```python
from build123d import *

# Parameters (mm, degrees)
F1_DEPTH  = 15
F2_W      = 3
F2_H      = 296.3
F3_DEPTH  = 25
F4_R      = 2.5
F5_DEPTH  = 3
F6_W      = 1
F6_H      = 0.5
F7_DEPTH  = 3
F8_R      = 1
F9_R      = 2.5
F9_R_2    = 1.2
F10_DEPTH = 3
F11_R     = 1.2
F12_DEPTH = 34.2
F13_DEPTH = 3
F14_R     = 2


with BuildPart() as f1:
    # F0 (on Right) → F1 (new body)
    with BuildSketch(Plane.YZ):
        Polygon((-7.5968508422, 3), (-7.5968508422, 0), (22.4031491578, 0), (22.4031491578, 304.3), (19.4031491578, 304.3), (19.4031491578, 3), align=None)
    extrude(amount=F1_DEPTH)

    # F2 (on face) → F3 (join)
    with BuildSketch(Plane(origin=(0, 22.4031491578, 0), x_dir=(-1, 0, 0), z_dir=(0, 1, 0))):
        with Locations((1.5, 156.15)):
            Rectangle(F2_W, F2_H)
        with Locations((-16.5, 156.15)):
            Rectangle(F2_W, F2_H)
    extrude(amount=-F3_DEPTH)

    # F4 (on face) → F5 (cut)
    with BuildSketch(Plane.XY.offset(3)):
        with Locations((7.5, -2.5968508422)):
            Circle(F4_R)
        with Locations((7.5, 12.4031491578)):
            Circle(F4_R)
    extrude(amount=-F5_DEPTH, mode=Mode.SUBTRACT)

    # F6 (on face) → F7 (cut)
    with BuildSketch(Plane.XZ.offset(-19.4031491578)):
        with Locations((0.5, 7.75)):
            Rectangle(F6_W, F6_H)
        with Locations((14.5, 7.75)):
            Rectangle(F6_W, F6_H)
    extrude(amount=-F7_DEPTH, mode=Mode.SUBTRACT)

    # F8
    f8_edges = [f1.edges().sort_by_distance(p)[0] for p in [
        (7.5, 19.403149, 3),
        (7.5, 22.403149, 0),
        (0, 19.403149, 156.15),
        (-3, 22.403149, 156.15),
        (18, 22.403149, 156.15),
        (15, 19.403149, 156.15),
    ]]
    fillet(f8_edges, radius=F8_R)

    # F9 (on face) → F10 (cut)
    with BuildSketch(Plane.XZ.offset(-19.4031491578)):
        with Locations((7.5, 298.3)):
            Circle(F9_R)
        with Locations((7.5, 100)):
            Circle(F9_R_2)
        with Locations((7.5, 200)):
            Circle(F9_R_2)
    extrude(amount=-F10_DEPTH, mode=Mode.SUBTRACT)

    # F11 (on face) → F12 (cut)
    with BuildSketch(Plane(origin=(-3, 0, 0), x_dir=(0, -1, 0), z_dir=(-1, 0, 0))):
        with Locations((-12.4031491578, 200)):
            Circle(F11_R)
        with Locations((-12.4031491578, 100)):
            Circle(F11_R)
        with Locations((-12.4031491578, 300)):
            Circle(F11_R)
    extrude(amount=-F12_DEPTH, mode=Mode.SUBTRACT)

    # F13 (add, symmetric): faces of the model
    f13_faces = [f1.faces().sort_by_distance(p)[0] for p in [
        (0, 9.1577983799, 1.9953507779),
        (15, 9.1577983799, 1.9953507779),
    ]]
    extrude(f13_faces, amount=F13_DEPTH, both=True, dir=(-1, 0, 0))

    # F14
    f14_edges = [f1.edges().sort_by_distance(p)[0] for p in [
        (-3, -7.596851, 1.5),
        (18, -7.596851, 1.5),
        (16.5, -2.596851, 8),
        (-1.5, -2.596851, 8),
        (-1.5, -2.596851, 304.3),
        (16.5, -2.596851, 304.3),
    ]]
    fillet(f14_edges, radius=F14_R)


solid = f1.part
```
Geometry check sheet. Reference: the model listing, model coordinates, mm. A direction names the side the tool comes from. Coordinates: 2 decimals unless noted, no trailing zeros. Order: outer loops, then holes, each group sorted by start corner. A loop starts at its lowest first (then second) coordinate and runs counter-clockwise, first axis right, second up. Notation, with made-up numbers: M 77.5,34.25 L 129.5,34.25 A25 cw 129.5,47.25 Z; hole C 29.5,-4.5 d6. An arc over 180 degrees is marked long. Answer as a JSON object with one key per item and string values.
Q1. Depth check by flat-ended pin: pin 1 Ø6 at (x, z) = (7.5, 298.3) entering from +Y; pin 2 Ø0.9 at (x, z) = (-1, 191.5) entering from -Y; pin 3 Ø3 at (x, y) = (12, -0.5) entering from +Z; pin 4 Ø3 at (x, y) = (7.5, -2.6) entering from -Z. Enter the tip coordinate at first touch or a pass-through.
Results are:
{"pin 1": "stops at y = 22.4", "pin 2": "stops at y = -2.6", "pin 3": "stops at z = 3", "pin 4": "passes through"}
Q2. Tool access check on faces 5 (the flat face through (7, 7, 0)), 6 (the flat face through (15, 8, 154)). Record the directions out of +Z, -Z, +X, -X, +Y, -Y that give a thin tool (end or side, any length) a straight path to the whole face; none if there is none.
Results are:
{"face 5": "-Z, +X, -X, +Y, -Y", "face 6": "+Z, -Y"}
Q3. Release check for a two-part mould opening along Y. For faces 1 (the cylindrical face through (9.885, -1.846, 1.521)), 2 (the flat face through (8, 22.403, 155)), 3 (the flat face through (7, 19.403, 156)), 4 (the flat face through (7, 6, 3)) record: released by +Y, released by -Y, zero draft, split by the parting line, or undercut.
Results are:
{"face 1": "undercut", "face 2": "released by +Y", "face 3": "released by -Y", "face 4": "zero draft"}
Q4. Scan lines: line 1 (Z direction, x = 7.5, y = 20.1); line 2 (Y direction, x = 7.5, z = 1.45); line 3 (X direction, y = 16, z = 160.5). Record each from-to range of solid material in increasing order.
Results are:
{"line 1": "z = 0 to 98.8, 101.2 to 198.8, 201.2 to 295.8, 300.8 to 304.3", "line 2": "y = -7.6 to -5.1, -0.1 to 9.9, 14.9 to 22.4", "line 3": "x = -3 to 0, 15 to 18"}
Q5. Cross-section at A-A on z = 40. Record the cut outline in (x, y).
Results are:
{"outline": "M -3,-2.6 L 0,-2.6 L 0,18.4 A1 cw 1,19.4 L 14,19.4 A1 cw 15,18.4 L 15,-2.6 L 18,-2.6 L 18,21.4 A1 ccw 17,22.4 L -2,22.4 A1 ccw -3,21.4 Z"}
